```python
from build123d import *

# Parameters (mm, degrees)
F3_DEPTH = 141.001


with BuildPart() as f1:
    # F0 (on Top) → F1 (revolve)
    with BuildSketch(Plane.XY):
        with BuildLine():
            Line((-68.743618687, 4.225), (-68.743618687, 0))
            Line((-68.743618687, 0), (70.256381313, 0))
            Line((70.256381313, 0), (72.256381313, 0))
            ThreePointArc((72.256381313, 0), (72.0293890684, 0.5480077554), (71.481381313, 0.775))
            Line((71.481381313, 0.775), (70.256381313, 0.775))
            Line((70.256381313, 0.775), (70.256381313, 1.5))
            Line((70.256381313, 1.5), (60.256381313, 4.225))
            Line((60.256381313, 4.225), (-18.9439036584, 4.225))
            Line((-18.9439036584, 4.225), (-18.9439036584, 3.725))
            Line((-18.9439036584, 3.725), (-19.1439036584, 3.725))
            Line((-19.1439036584, 3.725), (-19.1439036584, 4.225))
            Line((-19.1439036584, 4.225), (-61.5436239102, 4.225))
            Line((-61.5436239102, 4.225), (-61.5436239102, 3.003958482))
            Line((-61.5436239102, 3.003958482), (-63.043618687, 3))
            Line((-63.043618687, 3), (-63.043618687, 4.225))
            Line((-63.043618687, 4.225), (-68.743618687, 4.225))
        make_face()
    revolve(axis=Axis((0.756381313, 0, 0), (1, 0, 0)))

    # F2 (on face) → F3 (cut, through all)
    with BuildSketch(Plane(origin=(-68.743618687, 0, 0), x_dir=(0, -1, 0), z_dir=(-1, 0, 0))):
        with BuildLine():
            Line((-3, -2.975), (-3, 2.975))
            ThreePointArc((-3, 2.975), (-4.225, 0), (-3, -2.975))
        make_face()
        with BuildLine():
            ThreePointArc((4.225, 0), (3.9067649661, 1.6086679272), (3, 2.975))
            Line((3, 2.975), (3, -2.975))
            ThreePointArc((3, -2.975), (3.9067649661, -1.6086679272), (4.225, 0))
        make_face()
    extrude(amount=-F3_DEPTH, mode=Mode.SUBTRACT)


solid = f1.part
```
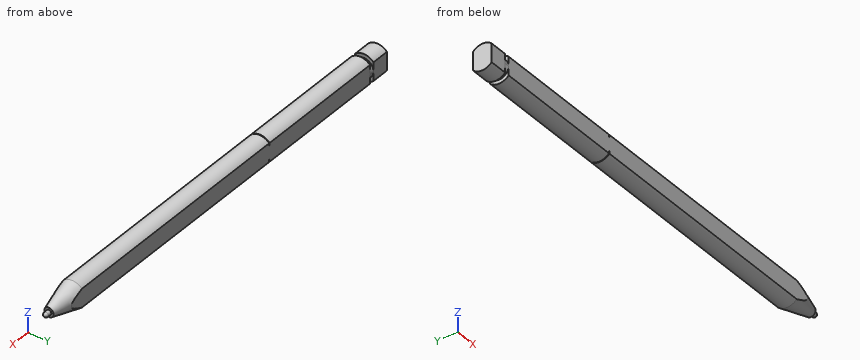
Part model, mm, in its own coordinate system. Coordinates: 2 decimals unless noted, no trailing zeros. Order: outer loops, then holes, each group sorted by start corner. A loop starts at its lowest first (then second) coordinate and runs counter-clockwise, first axis right, second up. Notation, with made-up numbers: (84, 79.5) - (141, 79.5) arc R11 ccw to (141, 94.5) - close; hole circle Ø10 at (-29.75, -26). An arc over 180 degrees is marked (long way). Return JSON: item names as keys, results as strings. Group by question number.
Item 1: Drill centre lines: probe 1 along Z at (x, y) = (24, -0.25); probe 2 along Z at (x, y) = (-48.5, -2); probe 3 along X at (y, z) = (-1, -0.25). Where is each one in solid material? Low to high. Write a range as from..to.
Item 2: Pin check, flat tip, straight feed: pin 1 (1.3 mm diameter, centred on y = 0, z = -2, fed in from +X). Stop position of the tip, or through.
Item 3: Cut at A-A (x = -42.5). List the corners of the cut face in (y, z) (3 decimals), plus the area to 3 significant figures.
Check values:
{
 "1": {"probe 1": "z = -4.22..4.22", "probe 2": "z = -3.72..3.72", "probe 3": "x = -68.74..70.26"},
 "2": {"pin 1": "stops at x = 70.26"},
 "3": {"outline": "(-3, -2.975) arc R4.225 ccw to (3, -2.975) - (3, 2.975) arc R4.225 ccw to (-3, 2.975) - close", "area": "46.0 mm2"}
}
